```python
from build123d import *

# Parameters (mm, degrees)
F1_DEPTH  = 25.4
F3_DEPTH  = 5.08
F5_DEPTH  = 5.08
F7_DEPTH  = 80.913372
F8_R      = 2.847327
F9_DEPTH  = 80.913372
F11_DEPTH = 25.4
F12_DEPTH = 25.4


with BuildPart() as f1:
    # F0 (on Top) → F1 (new body)
    with BuildSketch(Plane.XY):
        with BuildLine():
            Line((29.77816, 28.875791), (-30.379737, 28.875791))
            ThreePointArc((-30.379737, 28.875791), (-51.134211, 8.121316), (-30.379737, -12.633159))
            Line((-30.379737, -12.633159), (29.77816, -12.633159))
            ThreePointArc((29.77816, -12.633159), (50.532635, 8.121316), (29.77816, 28.875791))
        make_face()
    extrude(amount=F1_DEPTH)

    # F2 (on Front) → F3 (join)
    with BuildSketch(Plane.XZ):
        with BuildLine():
            Line((-30.379737, 59.542328), (-30.379737, 25.4))
            Line((-30.379737, 25.4), (29.77816, 25.4))
            Line((29.77816, 25.4), (29.77816, 59.542328))
            Line((29.77816, 59.542328), (15.948839, 59.542328))
            ThreePointArc((15.948839, 59.542328), (-0.531627, 43.41897), (-17.012093, 59.542328))
            Line((-17.012093, 59.542328), (-30.379737, 59.542328))
        make_face()
    extrude(amount=-F3_DEPTH)

    # F4 (on face) → F5 (join)
    with BuildSketch(Plane.XZ):
        with BuildLine():
            Line((-30.379737, 59.542328), (-30.379737, 25.4))
            Line((-30.379737, 25.4), (29.77816, 25.4))
            Line((29.77816, 25.4), (29.77816, 59.542328))
            Line((29.77816, 59.542328), (15.948839, 59.542328))
            ThreePointArc((15.948839, 59.542328), (-0.531627, 43.41897), (-17.012093, 59.542328))
            Line((-17.012093, 59.542328), (-30.379737, 59.542328))
        make_face()
    extrude(amount=F5_DEPTH)

    # F6 (on face) → F7 (cut, through all)
    with BuildSketch(Plane.YZ.offset(29.77816)):
        with BuildLine():
            Line((5.08, 51.302094), (5.08, 59.542328))
            Line((5.08, 59.542328), (-5.08, 59.542328))
            Line((-5.08, 59.542328), (-5.08, 51.567905))
            ThreePointArc((-5.08, 51.567905), (0.129474, 56.383832), (5.08, 51.302094))
        make_face()
    extrude(amount=-F7_DEPTH, mode=Mode.SUBTRACT)

    # F8 (on face) → F9 (cut, through all)
    with BuildSketch(Plane.YZ.offset(29.77816)):
        with Locations((-0.003477, 51.302094)):
            Circle(F8_R)
    extrude(amount=-F9_DEPTH, mode=Mode.SUBTRACT)

    # F10 (on Front) → F11 (cut)
    with BuildSketch(Plane.XZ):
        with BuildLine():
            Line((16.466387, 42.275124), (16.466387, 56.385571))
            Line((16.466387, 56.385571), (-16.873172, 56.385571))
            Line((-16.873172, 56.385571), (-16.873172, 44.329444))
            ThreePointArc((-16.873172, 44.329444), (-0.983531, 30.641417), (16.466387, 42.275124))
        make_face()
    extrude(amount=F11_DEPTH, mode=Mode.SUBTRACT)

    # F10 (on Front) → F12 (cut)
    with BuildSketch(Plane.XZ):
        with BuildLine():
            Line((16.466387, 42.275124), (16.466387, 56.385571))
            Line((16.466387, 56.385571), (-16.873172, 56.385571))
            Line((-16.873172, 56.385571), (-16.873172, 44.329444))
            ThreePointArc((-16.873172, 44.329444), (-0.983531, 30.641417), (16.466387, 42.275124))
        make_face()
    extrude(amount=-F12_DEPTH, mode=Mode.SUBTRACT)


solid = f1.part
```
Source: CAD feature listing. Evaluate the final solid. Frame: model axes, mm. A direction names the side the tool comes from. Coordinates: 2 decimals unless noted, no trailing zeros. Loops run counter-clockwise (first coordinate to the right, second up) from the corner with the lowest first, then second, coordinate; pieces in that order, holes last. Notation, with made-up numbers: (-35.5, 50.5) - (6.5, 50.5) arc R25 ccw to (6.5, 87.5) - close; hole circle Ø3 at (-17, 9). An arc over 180 degrees is marked (long way). Answer as CSV lines item,"result".
1. Reachability of faces 1 (the flat face through (-1, 5.08, 30)), 2 (the flat face through (29.778, 0, 41)), 3 (the flat face through (16.466, 0, 48)), 4 (the flat face through (0, 28.876, 13)), 5 (the cylindrical face through (23.215, 0.02, 56.386)) from +Z, -Z, +X, -X, +Y, -Y: full face, straight path, thin tool, end or side. Return the list, or none.
Established:
face 1,"+Z, +X, -X, +Y"
face 2,"+Z, +X, +Y, -Y"
face 3,"+Z, +Y, -Y"
face 4,"+Z, -Z, +X, -X, +Y"
face 5,"+Z, +X, -X"
2. Section C-C (y = -0.5). Return loops of the section in (x, z), then the cut area to 3 significant figures.
Established:
outline,"(-49.26, 0) - (48.66, 0) - (48.66, 25.4) - (29.78, 25.4) - (29.78, 48.5) - (16.47, 48.5) - (16.47, 42.28) arc R17.34 cw to (-16.87, 44.33) - (-16.87, 48.5) - (-30.38, 48.5) - (-30.38, 25.4) - (-49.26, 25.4) - close; (-30.38, 54.11) - (-16.87, 54.11) - (-16.87, 56.36) - (-30.38, 56.36) - close; (16.47, 54.11) - (29.78, 54.11) - (29.78, 56.36) - (16.47, 56.36) - close"
area,"3,450 mm2"
3. Contact query for flat-ended pins moving along their axis: pin 1 (4 mm diameter, centred on y = 11.5, z = 17.5, fed in from +X); pin 2 (3 mm diameter, centred on y = 1.5, z = 42, fed in from +X); pin 3 (5 mm diameter, centred on y = 2, z = 51.5, fed in from -X). Output: stop coordinate, or through.
Established:
pin 1,"stops at x = 50.49"
pin 2,"stops at x = 29.78"
pin 3,"stops at x = -30.38"
4. Mould query, pull axis X, two halves, no side actions, for faces 6 (the flat face through (-16.873, 0, 48)), 7 (the flat face through (-30.38, 0, 41)), 8 (the flat face through (-1, -5.08, 30)). Classes: released by +X, released by -X, zero draft, split by the parting line, or undercut.
Established:
face 6,"undercut"
face 7,"released by -X"
face 8,"zero draft"
5. Ray query, line 1 (X direction, y = 9, z = 8); line 2 (Z direction, x = 16, y = 10); line 3 (Z direction, x = -29, y = -1.5). Return the intervals inside material, ascending.
Established:
line 1,"x = -51.12 to 50.51"
line 2,"z = 0 to 25.4"
line 3,"z = 0 to 48.88, 53.72 to 56.16"
6. Section B-B (z = 32). Return loops of the section in (x, y), then the cut area to 3 significant figures.
Established:
outline,"(-30.38, -5.08) - (-6.72, -5.08) - (-6.72, 5.08) - (-30.38, 5.08) - close; (6.89, -5.08) - (29.78, -5.08) - (29.78, 5.08) - (6.89, 5.08) - close"
area,"473 mm2"
7. Section A-A (x = -20). Return loops of the section in (y, z).
Established:
outline,"(-12.63, 0) - (28.88, 0) - (28.88, 25.4) - (5.08, 25.4) - (5.08, 51.3) arc R5.08 ccw to (-5.08, 51.57) - (-5.08, 25.4) - (-12.63, 25.4) - close; hole circle Ø5.69 at (0, 51.3)"
8. Section D-D (x = -7.5). Return loops of the section in (y, z).
Established:
outline,"(-12.63, 0) - (28.88, 0) - (28.88, 25.4) - (5.08, 25.4) - (5.08, 32.35) - (-5.08, 32.35) - (-5.08, 25.4) - (-12.63, 25.4) - close"
